Verification items for the finished model (mm, model axes). Face numbers are marked on the shaded views. A direction names the side the tool comes from. Round coordinates to 2 decimals unless told otherwise and drop trailing zeros. Order: outer loops, then holes, each group sorted by start corner. A loop starts at its lowest first (then second) coordinate and runs counter-clockwise, first axis right, second up. Notation, with made-up numbers: M 51.25,7.25 L 85.25,7.25 A11 cw 85.25,25.25 Z; hole C 42,18.5 d11. An arc over 180 degrees is marked long. Return JSON: item names as keys, results as strings. Group by question number.
from build123d import *

# Parameters (mm, degrees)
SKETCH1_R           = 1.5
BOSS_EXTRUDE1_DEPTH = 35
SKETCH2_R           = 3
BOSS_EXTRUDE2_DEPTH = 3
FILLET1_R           = 1


with BuildPart() as part:
    # Sketch1 → Boss-Extrude1 (new body)
    with BuildSketch(Plane.XY):
        Circle(SKETCH1_R)
    extrude(amount=-BOSS_EXTRUDE1_DEPTH)

    # Sketch2 → Boss-Extrude2 (add)
    with BuildSketch(Plane.XY):
        Circle(SKETCH2_R)
    extrude(amount=BOSS_EXTRUDE2_DEPTH)

    # Fillet1
    fillet1_edges = [part.edges().sort_by_distance(p)[0] for p in [
        (-3, 0, 3),
    ]]
    fillet(fillet1_edges, radius=FILLET1_R)


solid = part.part
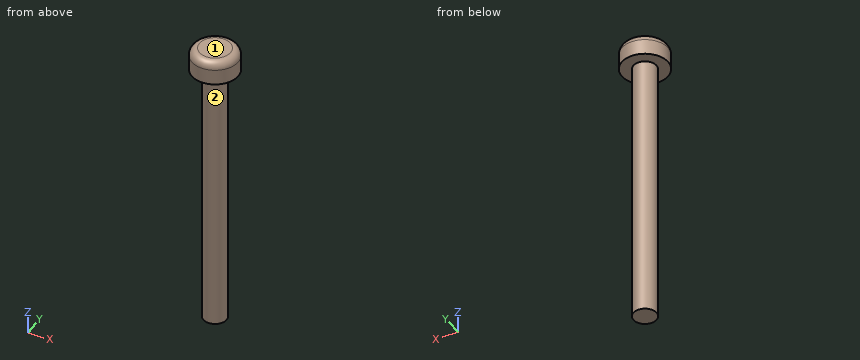
1. Thickness scan on line 1 along Z through (x, y) = (1.75, 0.55); line 2 along Y through (x, z) = (0.95, -4); line 3 along X through (y, z) = (-1.35, -31.5). Record the ranges inside material, lowest first. Write a range as from..to.
2. Go/stop test with flat-tipped pins: pin 1 (3 mm diameter, centred on x = -1.5, z = -3.5, fed in from +Y); pin 2 (2 mm diameter, centred on x = -0.5, z = -3.5, fed in from -Y). Record where each tip stops, or that it passes through.
3. Cross-section at C-C (z = -25). Enter the section's corners in (x, y).
4. Access from +Z, -Z, +X, -X, +Y, -Y to the whole of each face (thin tool, end or side, straight path). Record for the marked faces 1 and 2.
5. Cross-section at A-A (y = 0). Enter the section's corners in (x, z).
Computed:
{
 "1": {"line 1": "z = 0..3", "line 2": "y = -1.16..1.16", "line 3": "x = -0.65..0.65"},
 "2": {"pin 1": "stops at y = 1.5", "pin 2": "stops at y = -1.5"},
 "3": {"outline": "C 0,0 d3"},
 "4": {"face 1": "+Z, +X, -X, +Y, -Y", "face 2": "-Z"},
 "5": {"outline": "M -3,0 L -1.5,0 L -1.5,-35 L 1.5,-35 L 1.5,0 L 3,0 L 3,2 A1 ccw 2,3 L -2,3 A1 ccw -3,2 Z"}
}
